Check sheet for the modelled part. Datum: model origin and axes. Units: mm. Coordinates: 2 decimals unless noted, no trailing zeros. Loops run counter-clockwise (first coordinate to the right, second up) from the corner with the lowest first, then second, coordinate; pieces in that order, holes last.
```python
from build123d import *

# Parameters (mm, degrees)
SKETCH1_R           = 2.65
SKETCH1_R_2         = 7.5
BOSS_EXTRUDE2_DEPTH = 14


with BuildPart() as part:
    # Sketch1 → Boss-Extrude2 (new body)
    # profile 1 of 17: a face of its own
    with BuildSketch(Plane(origin=(0, 0, 0), x_dir=(1, 0, 0), z_dir=(0, 1, 0))):
        with BuildLine():
            ThreePointArc((54.623301063, -191.851720312), (51.393371136, -195.715064378), (51.3348715, -200.750384875))
            ThreePointArc((51.3348715, -200.750384875), (59.663021267, -205.712476174), (65.928383174, -198.314796214))
            ThreePointArc((65.928383174, -198.314796214), (65.928340244, -198.289420057), (65.928211455, -198.26404419))
            Line((65.928211455, -198.26404419), (62.928383174, -192.314796214))
            ThreePointArc((62.928383174, -192.314796214), (58.845920647, -190.826427737), (54.623301063, -191.851720312))
        make_face()
        with Locations(Location((58.428383174, -198.314796214, 0), (0, 0, 270))):
            Circle(SKETCH1_R, mode=Mode.SUBTRACT)
    # profile 2 of 17: a face of its own
    with BuildSketch(Plane(origin=(0, 0, 0), x_dir=(1, 0, 0), z_dir=(0, 1, 0))):
        with BuildLine():
            ThreePointArc((18.785357114, -87.475772959), (13.863470513, -86.411391053), (10.724167872, -82.474049884))
            Line((10.724167872, -82.474049884), (51.3348715, -200.750384875))
            ThreePointArc((51.3348715, -200.750384875), (51.393371136, -195.715064378), (54.623301063, -191.851720312))
            Line((54.623301063, -191.851720312), (18.785357114, -87.475772959))
        make_face()
    # profile 3 of 17: a face of its own
    with BuildSketch(Plane(origin=(0, 0, 0), x_dir=(1, 0, 0), z_dir=(0, 1, 0))):
        with BuildLine():
            ThreePointArc((14.012597561, -73.575385689), (10.782667702, -77.438729573), (10.724167872, -82.474049884))
            ThreePointArc((10.724167872, -82.474049884), (13.863470513, -86.411391053), (18.785357114, -87.475772959))
            Line((18.785357114, -87.475772959), (17.1084173, -82.591782349))
            ThreePointArc((17.1084173, -82.591782349), (15.311305548, -80.899036252), (15.689537375, -78.459376299))
            Line((15.689537375, -78.459376299), (14.012597561, -73.575385689))
        make_face()
    # profile 4 of 17: a face of its own
    with BuildSketch(Plane(origin=(0, 0, 0), x_dir=(1, 0, 0), z_dir=(0, 1, 0))):
        with BuildLine():
            ThreePointArc((25.317679673, -80.038461592), (21.540036733, -73.527389644), (14.012597561, -73.575385689))
            Line((14.012597561, -73.575385689), (15.689537375, -78.459376299))
            ThreePointArc((15.689537375, -78.459376299), (18.649221287, -77.522306083), (20.467679673, -80.038461592))
            ThreePointArc((20.467679673, -80.038461592), (19.421262336, -82.148206279), (17.1084173, -82.591782349))
            Line((17.1084173, -82.591782349), (18.785357114, -87.475772959))
            ThreePointArc((18.785357114, -87.475772959), (23.452729842, -84.987826157), (25.317679673, -80.038461592))
        make_face()
    # profile 5 of 17: a face of its own
    with BuildSketch(Plane(origin=(0, 0, 0), x_dir=(1, 0, 0), z_dir=(0, 1, 0))):
        with BuildLine():
            ThreePointArc((14.012597561, -73.575385689), (10.782667702, -77.438729573), (10.724167872, -82.474049884))
            ThreePointArc((10.724167872, -82.474049884), (13.863470513, -86.411391053), (18.785357114, -87.475772959))
            Line((18.785357114, -87.475772959), (17.1084173, -82.591782349))
            ThreePointArc((17.1084173, -82.591782349), (15.311305548, -80.899036252), (15.689537375, -78.459376299))
            Line((15.689537375, -78.459376299), (14.012597561, -73.575385689))
        make_face()
    # profile 6 of 17: a face of its own
    with BuildSketch(Plane(origin=(0, 0, 0), x_dir=(1, 0, 0), z_dir=(0, 1, 0))):
        with BuildLine():
            ThreePointArc((25.317679673, -80.038461592), (21.540036733, -73.527389644), (14.012597561, -73.575385689))
            Line((14.012597561, -73.575385689), (15.689537375, -78.459376299))
            ThreePointArc((15.689537375, -78.459376299), (18.649221287, -77.522306083), (20.467679673, -80.038461592))
            ThreePointArc((20.467679673, -80.038461592), (19.421262336, -82.148206279), (17.1084173, -82.591782349))
            Line((17.1084173, -82.591782349), (18.785357114, -87.475772959))
            ThreePointArc((18.785357114, -87.475772959), (23.452729842, -84.987826157), (25.317679673, -80.038461592))
        make_face()
    # profile 7 of 17: a face of its own
    with BuildSketch(Plane(origin=(0, 0, 0), x_dir=(1, 0, 0), z_dir=(0, 1, 0))):
        with BuildLine():
            ThreePointArc((5.146060616, -47.752107581), (0.22417418, -46.687725778), (-2.9151285, -42.750384875))
            Line((-2.9151285, -42.750384875), (10.724167872, -82.474049884))
            ThreePointArc((10.724167872, -82.474049884), (10.782667702, -77.438729573), (14.012597561, -73.575385689))
            Line((14.012597561, -73.575385689), (5.146060616, -47.752107581))
        make_face()
    # profile 8 of 17: a face of its own
    with BuildSketch(Plane(origin=(0, 0, 0), x_dir=(1, 0, 0), z_dir=(0, 1, 0))):
        with Locations((4.178383174, -40.314796214)):
            Circle(SKETCH1_R_2)
        with Locations(Location((4.178383174, -40.314796214, 0), (0, 0, 270))):
            Circle(SKETCH1_R, mode=Mode.SUBTRACT)
    # profile 9 of 17: a face of its own
    with BuildSketch(Plane(origin=(0, 0, 0), x_dir=(1, 0, 0), z_dir=(0, 1, 0))):
        with BuildLine():
            ThreePointArc((2.678383174, -5.663265443), (-1.631091845, -3.058212705), (-3.321616826, 1.685203786))
            Line((-3.321616826, 1.685203786), (-3.321616826, -40.314796214))
            ThreePointArc((-3.321616826, -40.314796214), (-1.631091845, -35.571379724), (2.678383174, -32.966326986))
            Line((2.678383174, -32.966326986), (2.678383174, -5.663265443))
        make_face()
    # profile 10 of 17: a face of its own
    with BuildSketch(Plane(origin=(0, 0, 0), x_dir=(1, 0, 0), z_dir=(0, 1, 0))):
        with Locations((4.178383174, 1.685203786)):
            Circle(SKETCH1_R_2)
        with Locations(Location((4.178383174, 1.685203786, 0), (0, 0, 270))):
            Circle(SKETCH1_R, mode=Mode.SUBTRACT)
    # profile 11 of 17: a face of its own
    with BuildSketch(Plane(origin=(0, 0, 0), x_dir=(1, 0, 0), z_dir=(0, 1, 0))):
        with BuildLine():
            ThreePointArc((14.332756859, 34.849450798), (11.140217836, 38.743750227), (11.130258872, 43.77940056))
            Line((11.130258872, 43.77940056), (-2.891321014, 4.189057352))
            ThreePointArc((-2.891321014, 4.189057352), (0.285789897, 8.095953943), (5.217707788, 9.112841657))
            Line((5.217707788, 9.112841657), (14.332756859, 34.849450798))
        make_face()
    # profile 12 of 17: a face of its own
    with BuildSketch(Plane(origin=(0, 0, 0), x_dir=(1, 0, 0), z_dir=(0, 1, 0))):
        with BuildLine():
            ThreePointArc((19.239287763, 48.703185114), (14.307369759, 47.686297331), (11.130258872, 43.77940056))
            ThreePointArc((11.130258872, 43.77940056), (11.140217836, 38.743750227), (14.332756859, 34.849450798))
            Line((14.332756859, 34.849450798), (16.056698099, 39.717049592))
            ThreePointArc((16.056698099, 39.717049592), (15.702001002, 42.160242169), (17.515346523, 43.835586319))
            Line((17.515346523, 43.835586319), (19.239287763, 48.703185114))
        make_face()
    # profile 13 of 17: a face of its own
    with BuildSketch(Plane(origin=(0, 0, 0), x_dir=(1, 0, 0), z_dir=(0, 1, 0))):
        with BuildLine():
            ThreePointArc((25.699963149, 41.275547242), (23.858802898, 46.197694406), (19.239287763, 48.703185114))
            Line((19.239287763, 48.703185114), (17.515346523, 43.835586319))
            ThreePointArc((17.515346523, 43.835586319), (19.813695769, 43.377538448), (20.849963149, 41.275547242))
            ThreePointArc((20.849963149, 41.275547242), (19.019367694, 38.755413081), (16.056698099, 39.717049592))
            Line((16.056698099, 39.717049592), (14.332756859, 34.849450798))
            ThreePointArc((14.332756859, 34.849450798), (21.890894795, 34.746609841), (25.699963149, 41.275547242))
        make_face()
    # profile 14 of 17: a face of its own
    with BuildSketch(Plane(origin=(0, 0, 0), x_dir=(1, 0, 0), z_dir=(0, 1, 0))):
        with BuildLine():
            ThreePointArc((19.239287763, 48.703185114), (14.307369759, 47.686297331), (11.130258872, 43.77940056))
            ThreePointArc((11.130258872, 43.77940056), (11.140217836, 38.743750227), (14.332756859, 34.849450798))
            Line((14.332756859, 34.849450798), (16.056698099, 39.717049592))
            ThreePointArc((16.056698099, 39.717049592), (15.702001002, 42.160242169), (17.515346523, 43.835586319))
            Line((17.515346523, 43.835586319), (19.239287763, 48.703185114))
        make_face()
    # profile 15 of 17: a face of its own
    with BuildSketch(Plane(origin=(0, 0, 0), x_dir=(1, 0, 0), z_dir=(0, 1, 0))):
        with BuildLine():
            ThreePointArc((25.699963149, 41.275547242), (23.858802898, 46.197694406), (19.239287763, 48.703185114))
            Line((19.239287763, 48.703185114), (17.515346523, 43.835586319))
            ThreePointArc((17.515346523, 43.835586319), (19.813695769, 43.377538448), (20.849963149, 41.275547242))
            ThreePointArc((20.849963149, 41.275547242), (19.019367694, 38.755413081), (16.056698099, 39.717049592))
            Line((16.056698099, 39.717049592), (14.332756859, 34.849450798))
            ThreePointArc((14.332756859, 34.849450798), (21.890894795, 34.746609841), (25.699963149, 41.275547242))
        make_face()
    # profile 16 of 17: a face of its own
    with BuildSketch(Plane(origin=(0, 0, 0), x_dir=(1, 0, 0), z_dir=(0, 1, 0))):
        with BuildLine():
            ThreePointArc((51.311176885, 139.259107341), (48.118637818, 143.153406895), (48.108678986, 148.189057352))
            Line((48.108678986, 148.189057352), (11.130258872, 43.77940056))
            ThreePointArc((11.130258872, 43.77940056), (14.307369759, 47.686297331), (19.239287763, 48.703185114))
            Line((19.239287763, 48.703185114), (51.311176885, 139.259107341))
        make_face()
    # profile 17 of 17: a face of its own
    with BuildSketch(Plane(origin=(0, 0, 0), x_dir=(1, 0, 0), z_dir=(0, 1, 0))):
        with Locations((55.178383174, 145.685203786)):
            Circle(SKETCH1_R_2)
        with Locations(Location((55.178383174, 145.685203786, 0), (0, 0, 270))):
            Circle(SKETCH1_R, mode=Mode.SUBTRACT)
    extrude(amount=BOSS_EXTRUDE2_DEPTH)


solid = part.part
```
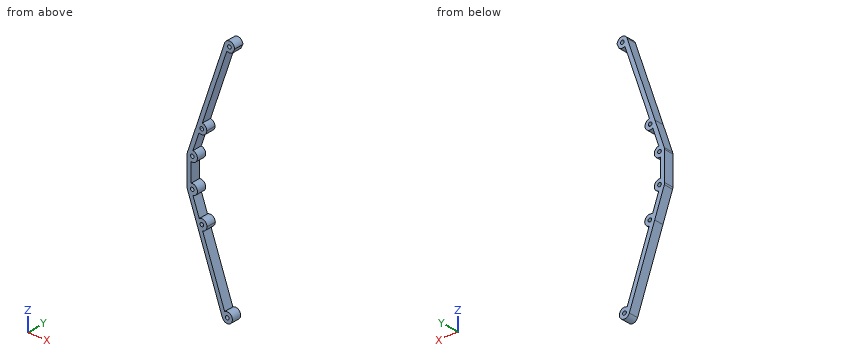
1) Section check D-D on z = -59.5. Enter the section's corners in (x, y).
Answer sheet:
outline: (16.7, 0) - (23.06, 0) - (23.06, 14) - (16.7, 14) - close
2) Scan lines: line 1 (Z direction, x = 58.5, y = 12.25); line 2 (Z direction, x = 56, y = 11.25); line 3 (X direction, y = 7.5, z = 15). Record each from-to range of solid material in increasing order.
Answer sheet:
line 1: z = -152.41 to -138.96, 190.82 to 195.67, 200.96 to 205.81
line 2: z = -153.14 to -148.2, -143.17 to -138.23, 191.22 to 197.25, 199.38 to 205.41
line 3: x = -3.32 to 2.68
3) Depth check by flat-ended pin: pin 1 (5 mm diameter, centred on y = 4.5, z = 12.5, fed in from +X); pin 2 (1 mm diameter, centred on x = 55.5, y = 6, fed in from -Z); pin 3 (3 mm diameter, centred on x = 4.18, z = 40.31, fed in from +Y); pin 4 (3 mm diameter, centred on y = 7.5, z = -49, fed in from -X). Enter the tip coordinate at first touch or a pass-through.
Answer sheet:
pin 1: stops at x = 2.68
pin 2: stops at z = -153.19
pin 3: passes through
pin 4: stops at x = 12.45
4) Section check C-C on z = 12.5. Enter the section's corners in (x, y).
Answer sheet:
outline: (-3.32, 0) - (2.68, 0) - (2.68, 14) - (-3.32, 14) - close
5) Section check B-B on x = 31. Enter the section's corners in (y, z), plus the area to 3 significant figures.
Answer sheet:
outline: (0, -99.88) - (14, -99.88) - (14, -81.91) - (0, -81.91) - close; (0, 123.05) - (14, 123.05) - (14, 141.53) - (0, 141.53) - close
area: 510 mm2
6) Section check A-A on y = 8.5. Enter the section's corners in (x, z), plus the area to 3 significant figures.
Answer sheet:
outline: (-3.32, -1.69) arc R7.5 ccw to (-2.89, -4.19) - (48.11, -148.19) arc R7.5 ccw (long way) to (51.31, -139.26) - (19.24, -48.7) arc R7.5 ccw (long way) to (14.33, -34.85) - (5.22, -9.11) arc R7.5 ccw (long way) to (2.68, 5.66) - (2.68, 32.97) arc R7.5 ccw (long way) to (5.15, 47.75) - (14.01, 73.58) arc R7.5 ccw (long way) to (18.79, 87.48) - (54.62, 191.85) arc R7.5 ccw to (62.93, 192.31) - (65.93, 198.26) arc R7.5 ccw to (65.93, 198.31) arc R7.5 ccw to (51.33, 200.75) - (-2.92, 42.75) arc R7.5 ccw to (-3.32, 40.31) - close; hole circle Ø5.3 at (4.18, -1.69); hole circle Ø5.3 at (4.18, 40.31); hole circle Ø5.3 at (17.82, 80.04); hole circle Ø5.3 at (18.2, -41.28); hole circle Ø5.3 at (55.18, -145.69); hole circle Ø5.3 at (58.43, 198.31)
area: 2,770 mm2
